```python
from build123d import *


with BuildPart() as f1:
    # F0 (on Front) → F1 (revolve)
    with BuildSketch(Plane.XZ):
        Polygon((0, -212.00102), (0, -202.47602), (-101.6, -202.47602), (-101.6, 51.52398), (-136.525, 51.52398), (-136.525, 41.99898), (-111.125, 41.99898), (-111.125, -212.00102), align=None)
    revolve(axis=Axis((0, 0, -78.97687), (0, 0, -1)))

    # F4: sweep along a path in F2
    with BuildLine(Plane.XY.offset(51.52398)) as f4_path:
        CenterArc((0, 0), 123.825, 0, 360)
    # F3 (on Front) → F4 (sweep, cut)
    with BuildSketch(Plane.XZ):
        with BuildLine():
            Line((-121.1326, 51.52398), (-126.5174, 51.52398))
            ThreePointArc((-126.5174, 51.52398), (-123.825, 48.83158), (-121.1326, 51.52398))
        make_face()
    sweep(path=f4_path.line, mode=Mode.SUBTRACT)


solid = f1.part
```
CAD build for the part. Positions are in the model's coordinates, mm. A direction names the side the tool comes from. Round coordinates to 2 decimals unless told otherwise and drop trailing zeros. Order: outer loops, then holes, each group sorted by start corner. A loop starts at its lowest first (then second) coordinate and runs counter-clockwise, first axis right, second up. Notation, with made-up numbers: (-31, -37) -> (-20, -37) arc R25 ccw to (-20, -24) -> close; hole circle Ø5 at (-34, 61). An arc over 180 degrees is marked (long way). One line per question, with ' | ' between items.
Q1. Slice it at A-A (y = 0). Write the cut outline in (x, z) (3 decimals), then the cut area to 3 significant figures.
Completed:
outline: (-136.525, 41.999) -> (-111.125, 41.999) -> (-111.125, -212.001) -> (111.125, -212.001) -> (111.125, 41.999) -> (136.525, 41.999) -> (136.525, 51.524) -> (126.517, 51.524) arc R2.692 cw to (121.133, 51.524) -> (101.6, 51.524) -> (101.6, -202.476) -> (-101.6, -202.476) -> (-101.6, 51.524) -> (-121.133, 51.524) arc R2.692 cw to (-126.517, 51.524) -> (-136.525, 51.524) -> close | area: 7,420 mm^2
Q2. Two-plate mould, pull along Y, no slides. Class faces 4 (the cylindrical face through (136.393, 6.003, 46.695)), 5 (the flat face through (-1, 1, -202.476)), 6 (the flat face through (121, -40, 51.524)): released by +Y, released by -Y, zero draft, split by the parting line, or undercut.
Completed:
face 4: split by the parting line | face 5: undercut | face 6: zero draft
Q3. Drop flat-ended pins along their axis: pin 1 (3 mm diameter, centred on x = -41, y = -14, fed in from +Z); pin 2 (4 mm diameter, centred on x = 81.5, z = -122, fed in from -Y); pin 3 (5 mm diameter, centred on x = -50.5, z = -179, fed in from +Y). Give the stop position or say it passes through.
Completed:
pin 1: stops at z = -202.48 | pin 2: stops at y = -77.64 | pin 3: stops at y = 100.22
Q4. Probe probe 1 along Z at (x, y) = (-69, 107.5); probe 2 along Y at (x, z) = (0, -138.5) (3 decimals); probe 3 along Y at (x, z) = (69.5, -46). List the from-to ranges inside material, lowest first.
Completed:
probe 1: z = 42 to 51.52 | probe 2: y = -111.125 to -101.6, 101.6 to 111.125 | probe 3: y = -86.71 to -74.11, 74.11 to 86.71
Q5. Slice it at B-B (z = -25.5). Write the cut outline in (x, y) (3 decimals).
Completed:
outline: circle Ø222.25 at (0, 0); hole circle Ø203.2 at (0, 0)
Q6. Which spindle directions (+Z, -Z, +X, -X, +Y, -Y) get a long thin tool onto all of the face, cutting with end or side? Do faces 1 (the cylindrical face through (22.025, -99.184, -73.698)), 2 (the cylindrical face through (14.47, 110.18, -86.78)), 3 (the flat face through (2, 2, -212.001)). Say none if no direction does.
Completed:
face 1: +Z | face 2: -Z | face 3: -Z, +X, -X, +Y, -Y
